Work out the finished part from the listing and answer in its coordinate system (mm). Face numbers are marked on the shaded views. A direction names the side the tool comes from. Give positions to 0.01 mm unless a question says otherwise; leave off trailing zeros. Order: outer loops, then holes, each group sorted by start corner. A loop starts at its lowest first (then second) coordinate and runs counter-clockwise, first axis right, second up.
Solid Edge part; units mm, degrees
sketch "Sketch1" plane through (0, 0, 0) normal (1, 0, 0) x (0, 1, 0)
  circle A0 centre (0, 0) radius 3
extrude "Protrusion1" add sketch "Sketch1" along normal mid plane 7
sketch "Sketch2" plane through (-3.5, 0, 0) normal (-1, 0, 0) x (0, 1, 0)
  circle A0 centre (0, 0) radius 4
extrude "ExtrudedProtrusion_2" add sketch "Sketch2" against normal blind 2
sketch "Sketch3" plane through (3.5, 0, 0) normal (1, 0, 0) x (0, 1, 0)
  circle A0 centre (0, 0) radius 2.0005
extrude "ExtrudedCutout_1" cut sketch "Sketch3" along normal mid plane 52.3532
sketch "Sketch4" plane through (0, 0, 0) normal (0, 0, 1) x (1, 0, 0)
  circle A0 centre (1, 0) radius 1
extrude "ExtrudedCutout_2" cut sketch "Sketch4" along normal mid plane 12.1891
properties material "PVC"
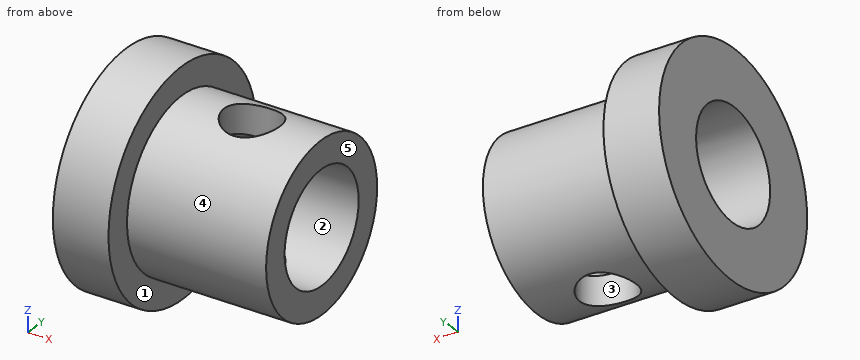
1. Given P1, Ø1.8, axis at x = 1, y = 0, coming from the +Z side; P2, Ø2.5, axis at y = -0.5, z = -1.5, coming from the +X side; P3, Ø1, axis at x = 0, y = -1.5, coming from the -Z side, each flat-ended and moving along its own axis, determine where each tip first touches the part or whether it passes through.
Findings below:
P1: passes through
P2: stops at x = 3.5
P3: stops at z = -2.83
2. The part is cut by section D-D (z = 2.75). Write down the section's boundary in (x, y), then the cut area to 3 significant figures.
Findings below:
outline: (-3.5, -2.9) - (-1.5, -2.9) - (-1.5, -1.2) - (3.5, -1.2) - (3.5, 1.2) - (-1.5, 1.2) - (-1.5, 2.9) - (-3.5, 2.9) - close; hole circle Ø2 at (1, 0)
area: 20.5 mm2
3. Straight lines are drawn through the part: probe 1 along X at (y, z) = (0, -2.55); probe 2 along Z at (x, y) = (-1.25, 0); probe 3 along X at (y, z) = (0.5, -2.5). For each, find the intervals that lie inside material, in ascending order.
Findings below:
probe 1: x = -3.5 to 0, 2 to 3.5
probe 2: z = -3 to -2, 2 to 3
probe 3: x = -3.5 to 0.13, 1.87 to 3.5
4. Which of the six approach directions +Z, -Z, +X, -X, +Y, -Y give full straight-line access (tool end or side, diameter ignored) to the marked faces 1 and 2?
Findings below:
face 1: +X
face 2: +X, -X
5. The part is cut by section B-B (z = 0). Write down the section's boundary in (x, y).
Findings below:
outline: (-3.5, -4) - (-1.5, -4) - (-1.5, -3) - (3.5, -3) - (3.5, -2) - (-3.5, -2) - close; (-3.5, 2) - (3.5, 2) - (3.5, 3) - (-1.5, 3) - (-1.5, 4) - (-3.5, 4) - close
6. The mould has two halves that part along Y. Classify the marked faces 3, 4 and 5: pulls with the +Y half, pulls with the -Y half, needs draft (parallel to the pull), parting line crosses it, or undercut.
Findings below:
face 3: undercut
face 4: parting line crosses it
face 5: needs draft
7. The part is cut by section A-A (y = 0). Write down the section's boundary in (x, z).
Findings below:
outline: (-3.5, -4) - (-1.5, -4) - (-1.5, -3) - (0, -3) - (0, -2) - (-3.5, -2) - close; (-3.5, 2) - (0, 2) - (0, 3) - (-1.5, 3) - (-1.5, 4) - (-3.5, 4) - close; (2, -3) - (3.5, -3) - (3.5, -2) - (2, -2) - close; (2, 2) - (3.5, 2) - (3.5, 3) - (2, 3) - close
8. The part is cut by section C-C (x = 0.75). Write down the section's boundary in (y, z).
Findings below:
outline: (-0.97, -2.84) - (-0.97, -1.75) arc R2 cw to (-0.97, 1.75) - (-0.97, 2.84) arc R3 ccw to start; (0.97, -2.84) arc R3 ccw to (0.97, 2.84) - (0.97, 1.75) arc R2 cw to (0.97, -1.75) - close
